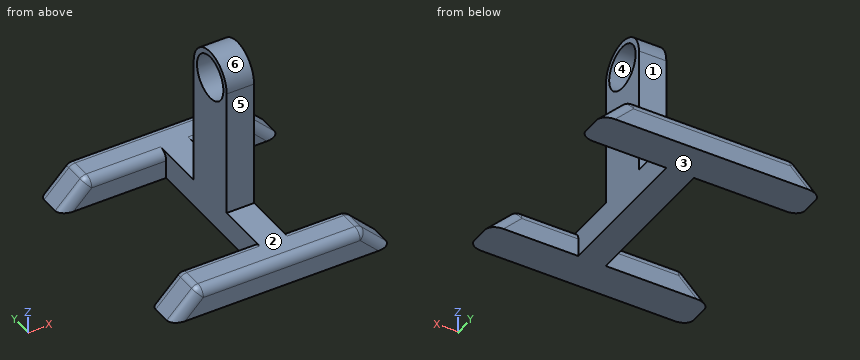
```python
from build123d import *

# Parameters (mm, degrees)
F1_DEPTH  = 20
F2_W      = 15
F2_H      = 15
F3_DEPTH  = 80
F4_W      = 15
F4_H      = 15
F5_DEPTH  = 20
F6_R      = 5
F8_DEPTH  = 85
F10_DEPTH = 25
F11_R     = 12
F12_DEPTH = 72.7991883287


with BuildPart() as f1:
    # F0 (on Front) → F1 (new body)
    with BuildSketch(Plane.XZ):
        Polygon((-19.1690939665, 0), (-49.1690939665, 0), (-64.1690939665, 0), (-79.1690939665, -15), (-49.1690939665, -15), (10.8309060335, -15), (40.8309060335, -15), (25.8309060335, 0), (10.8309060335, 0), align=None)
    extrude(amount=F1_DEPTH)

    # F2 (on face) → F3 (join)
    with BuildSketch(Plane(origin=(0, 0, 0), x_dir=(-1, 0, 0), z_dir=(0, 1, 0))):
        with Locations((14.7267927229, -7.5)):
            Rectangle(F2_W, F2_H)
    extrude(amount=F3_DEPTH)

    # F4 (on face) → F5 (join)
    with BuildSketch(Plane(origin=(0, 80, 0), x_dir=(-1, 0, 0), z_dir=(0, 1, 0))):
        Polygon((7.2267927229, 0), (-24.975023807, 0), (-39.9750189483, -15), (-19.9750189483, -15), (7.2267927229, -15), align=None)
        with Locations((14.7267927229, -7.5)):
            Rectangle(F4_W, F4_H)
        Polygon((65.0249859104, 0), (22.2267927229, 0), (22.2267927229, -15), (60.0249810517, -15), (80.0249810517, -15), align=None)
    extrude(amount=F5_DEPTH)

    # F6
    f6_edges = [f1.edges().sort_by_distance(p)[0] for p in [
        (-65.024986, 90, 0),
        (24.975024, 90, 0),
        (-64.169094, -10, 0),
        (25.830906, -10, 0),
        (-43.197943, 0, 0),
        (9.302057, 0, 0),
        (33.330906, 0, -7.5),
        (-71.669094, 0, -7.5),
        (-71.669094, -20, -7.5),
        (-19.169094, -20, 0),
        (33.330906, -20, -7.5),
        (8.874116, 80, 0),
        (-43.625889, 80, 0),
        (-72.524983, 80, -7.5),
        (-72.524983, 100, -7.5),
        (-20.024981, 100, 0),
        (32.475021, 100, -7.5),
        (32.475021, 80, -7.5),
    ]]
    fillet(f6_edges, radius=F6_R)

    # F7 (on face) → F8 (join)
    with BuildSketch(Plane.XY):
        Polygon((-22.2267927229, 25), (-7.2267927229, 25), (-7.2267927229, 55), (-22.2267927229, 55), (-22.2267927229, 40), align=None)
    extrude(amount=F8_DEPTH)

    # F9 (on face) → F10 (cut)
    with BuildSketch(Plane.YZ.offset(-7.2267927229)):
        with BuildLine():
            ThreePointArc((25, 70), (29.3933982822, 80.6066017178), (40, 85))
            Line((40, 85), (25, 85))
            Line((25, 85), (25, 70))
        make_face()
        with BuildLine():
            Line((55, 85), (40, 85))
            ThreePointArc((40, 85), (50.6066017178, 80.6066017178), (55, 70))
            Line((55, 70), (55, 85))
        make_face()
    extrude(amount=-F10_DEPTH, mode=Mode.SUBTRACT)

    # F11 (on face) → F12 (cut, through all)
    with BuildSketch(Plane.YZ.offset(-7.2267927229)):
        with Locations((40, 70)):
            Circle(F11_R)
    extrude(amount=-F12_DEPTH, mode=Mode.SUBTRACT)


solid = f1.part
```
For this review, take the finished solid that the model builds, in its own axes (mm). Face numbers are marked on the shaded views. A direction names the side the tool comes from. Round coordinates to 2 decimals unless told otherwise and drop trailing zeros. Write each loop counter-clockwise with the first axis right and the second up, starting at its lowest first coordinate (ties: lowest second). Pieces come first, ordered by that corner, then holes. Notation, with made-up numbers: (-34.5, 58) - (-24.5, 58) arc R23 cw to (-24.5, 85) - close; hole circle Ø4 at (63, 20.5). An arc over 180 degrees is marked (long way). Answer as a JSON object with one key per item and string values.
1. For pin 1 Ø2 at (y, z) = (29, 21) entering from -X; pin 2 Ø3 at (x, y) = (-19.5, 68) entering from +Z; pin 3 Ø16.5 at (x, z) = (-15.5, 40) entering from -Y, all flat-tipped, find the tip position at first contact; note any pin that passes through.
Response values:
{"pin 1": "stops at x = -22.23", "pin 2": "stops at z = 0", "pin 3": "stops at y = 25"}
2. We need section A-A on x = -2. Give the boundary of the cut face in (y, z), then the cut area to 3 significant figures.
Response values:
{"outline": "(-20, -15) - (0, -15) - (0, -5) arc R5 ccw to (-5, 0) - (-15, 0) arc R5 ccw to (-20, -5) - close; (80, -15) - (100, -15) - (100, -5) arc R5 ccw to (95, 0) - (85, 0) arc R5 ccw to (80, -5) - close", "area": "579 mm2"}
3. We need section C-C on x = -20. Give the boundary of the cut face in (y, z).
Response values:
{"outline": "(-20, -15) - (100, -15) - (100, -5) arc R5 ccw to (95, 0) - (55, 0) - (55, 70) arc R15 ccw to (25, 70) - (25, 0) - (-15, 0) arc R5 ccw to (-20, -5) - close; hole circle Ø24 at (40, 70)"}
4. Draft analysis for pull direction Z (two halves, no side actions). For the marked faces 4, 5 and 6, state which applies: +Z half, -Z half, draft (parallel to the pull), parting line (faces both ways), or undercut.
Response values:
{"face 4": "undercut", "face 5": "draft", "face 6": "+Z half"}
5. We need section B-B on y = 40. Give the boundary of the cut face in (x, z).
Response values:
{"outline": "(-22.23, -15) - (-7.23, -15) - (-7.23, 58) - (-22.23, 58) - close; (-22.23, 82) - (-7.23, 82) - (-7.23, 85) - (-22.23, 85) - close"}
6. Tool access review of the marked faces 1, 2 and 3: name each direction out of +Z, -Z, +X, -X, +Y, -Y from which nothing blocks a thin tool from reaching the whole face with its end or side.
Response values:
{"face 1": "+Z, +X, -X, +Y", "face 2": "+Z, +X, -X, -Y", "face 3": "-Z, +X, -X, +Y, -Y"}
7. We need section D-D on z = 38. Give the boundary of the cut face in (x, y).
Response values:
{"outline": "(-22.23, 25) - (-7.23, 25) - (-7.23, 55) - (-22.23, 55) - close"}
8. To check wall thickness, follow line 1 along Z through (x, y) = (-16.25, 40); line 2 along Y through (x, z) = (-39, -9.5); line 3 along X through (y, z) = (36, 23). State the ranges of each line that lie inside material, in increasing order.
Response values:
{"line 1": "z = -15 to 58, 82 to 85", "line 2": "y = -20 to 0, 80 to 100", "line 3": "x = -22.23 to -7.23"}
